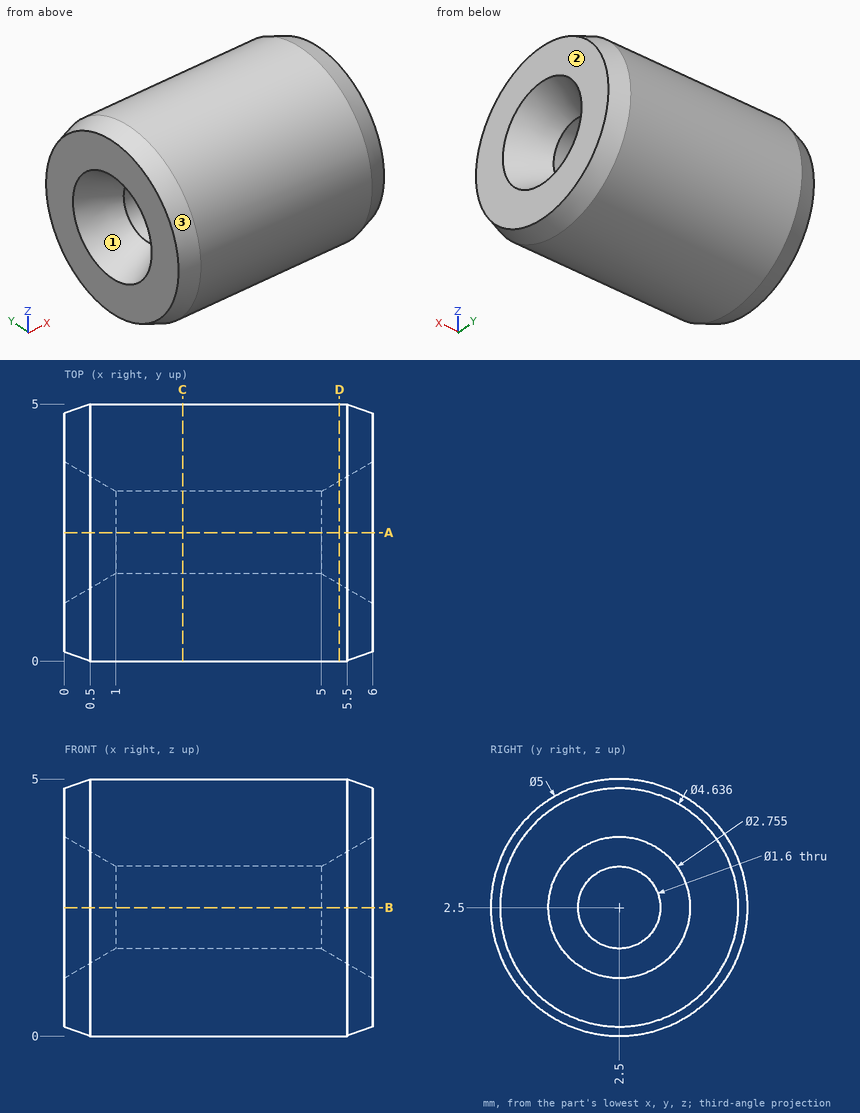
Part print with two shaded views. Sizes in mm from the minimum x, y, z corner. Give positions to 0.01 mm unless a question says otherwise; leave off trailing zeros. Loops run counter-clockwise (first coordinate to the right, second up) from the corner with the lowest first, then second, coordinate; pieces in that order, holes last. Notation, with made-up numbers: (-38.5, 47) -> (13.5, 47) arc R22 cw to (13.5, 76) -> close; hole circle Ø7 at (29.25, -30). An arc over 180 degrees is marked (long way). One line per question, with ' | ' between items.
Q1. Cut at A-A, the plane y = 2.5. Write the cut outline in (x, z).
Filled sheet:
outline: (0, 0.18) -> (0.5, 0) -> (5.5, 0) -> (6, 0.18) -> (6, 1.12) -> (5, 1.7) -> (1, 1.7) -> (0, 1.12) -> close; (0, 3.88) -> (1, 3.3) -> (5, 3.3) -> (6, 3.88) -> (6, 4.82) -> (5.5, 5) -> (0.5, 5) -> (0, 4.82) -> close
Q2. Drill centre lines: line 1 along Y through (x, z) = (0.85, 1.7) (1 decimal); line 2 along Z through (x, y) = (3.25, 3.15) (1 decimal); line 3 along Y through (x, z) = (0.8, 2.2) (1 decimal). Where is each one in solid material? Low to high. Write a range as [from, to].
Filled sheet:
line 1: y = [0.1, 2.1], [2.9, 4.9] | line 2: z = [0.1, 2], [3, 4.9] | line 3: y = [0, 1.6], [3.4, 5]
Q3. Drop a flat-ended pin along its axis: pin 1 (1.5 mm diameter, centred on x = 3.5, z = 3.5, fed in from -Y). Give the stop position or say it passes through.
Filled sheet:
pin 1: stops at y = 0.01
Q4. Pull direction Z, two halves, no side cores. Call the marked faces 1, 2 and 3: pulls with the +Z half, pulls with the -Z half, needs draft (parallel to the pull), parting line crosses it, or undercut.
Filled sheet:
face 1: undercut | face 2: needs draft | face 3: parting line crosses it
Q5. Cut at C-C, the plane x = 2.3. Write the cut outline in (y, z), plus the area to 3 significant figures.
Filled sheet:
outline: circle Ø5 at (2.5, 2.5); hole circle Ø1.6 at (2.5, 2.5) | area: 17.6 mm²
Q6. Cut at D-D, the plane x = 5.35. Write the cut outline in (y, z).
Filled sheet:
outline: circle Ø5 at (2.5, 2.5); hole circle Ø2 at (2.5, 2.5)
